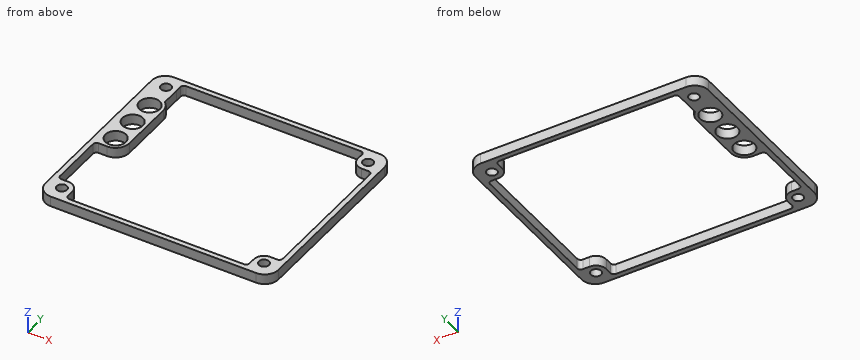
Autodesk Fusion 360 part; units mm, degrees
sketch "Sketch1" plane through (0, 0, 0) normal (0, 0, 1) x (1, 0, 0)
  line L0 (-29.5, 24.5) -> (-35.5, 24.5) construction
  circle A0 centre (29.5, 24.5) radius 1.5
  line L1 (25.5009, -27.5) -> (3.5, -27.5)
  arc A1 (34, 25) -> (30, 29) centre (30, 25) ccw
  circle A2 centre (29.5, -24.5) radius 1.5
  arc A3 (30, -29) -> (34, -25) centre (30, -25) ccw
  line L2 (30, -29) -> (-30, -29)
  arc A4 (-34, -25) -> (-30, -29) centre (-30, -25) ccw
  line L3 (0, -27.5) -> (0.5, -27.5) construction
  line L4 (0.5, -27.5) -> (-25.5, -27.5)
  line L5 (-30, 29) -> (30, 29)
  line L6 (0, 27.5) -> (0.5, 27.5) construction
  circle A5 centre (-29.5, 24.5) radius 1.5
  arc A6 (-30, 29) -> (-34, 25) centre (-30, 25) ccw
  line L7 (0, -27.5) -> (0.5, -27.5) construction
  line L8 (-34, -25) -> (-34, 25)
  circle A7 centre (-29.5, -24.5) radius 1.5
  line L9 (0, -27.5) -> (0.5, -27.5)
  line L10 (34, 25) -> (34, -25)
  line L11 (-29.5, 24.5) -> (-34, 24.5) construction
  line L12 (-34, 24.5) -> (-34, 29) construction
  line L13 (-34, 29) -> (-29.5, 29) construction
  line L14 (-29.5, 29) -> (-29.5, 24.5) construction
  line L15 (-34, 29) -> (-29, 29) construction
  line L16 (-29, 29) -> (-29, 16) construction
  line L17 (-29, 16) -> (-34, 16) construction
  line L18 (-34, 16) -> (-34, 29) construction
  line L19 (-25, 13) -> (-25, 11)
  line L20 (-25, 5) -> (-25, 3)
  line L21 (-25, 13) -> (-25, 16)
  line L22 (-25, 11) -> (-25, 5)
  line L23 (-25, 3) -> (-25, 0)
  line L24 (-26.5, 24.4915) -> (-26.494, 26.6091)
  line L25 (-26.5, 24.4915) -> (-26.5151, 19.1346)
  arc A8 (-25.5, 27.5) -> (-26.4946, 26.3966) centre (-25.5, 26.5) ccw
  line L26 (-30, 27.5) -> (-29, 27.5)
  line L27 (-25.5, 27.5) -> (0.5, 27.5)
  arc A9 (-29, 27.458) -> (-29.5, 27.5) centre (-29.5, 24.5) ccw
  arc A10 (-29, 27.458) -> (-29.5, 27.5) centre (-29.5, 24.5) ccw
  circle A11 centre (-29, 16) radius 3
  circle A12 centre (-29, 8) radius 3
  circle A13 centre (-29, 0) radius 3
  arc A14 (-25, 16) -> (-26.5151, 19.1346) centre (-29, 16) ccw
  arc A15 (-29, -4) -> (-25, 0) centre (-29, 0) ccw
  line L28 (-32.5, -20.5009) -> (-32.5, -4.999)
  line L29 (-29, -3) -> (-29, -4) construction
  line L30 (-29, -4) -> (-31.5, -4)
  line L31 (-29.5, -24.5) -> (-26.5, -24.5) construction
  line L32 (-26.5, -24.5) -> (-26.5, -21.5) construction
  line L33 (-26.5, -21.5) -> (-29.5, -21.5) construction
  line L34 (-29.5, -21.5) -> (-29.5, -24.5) construction
  line L35 (-26.5, -24.5) -> (-26.5, -26.5)
  line L36 (-29.5, -21.5) -> (-31.5, -21.5)
  arc A16 (-26.5, -24.5015) -> (-29.5014, -21.5) centre (-29.5, -24.5) ccw
  arc A17 (-31.5, -4) -> (-32.5, -5.001) centre (-31.5, -5) ccw
  arc A18 (-32.5, -20.4991) -> (-31.5, -21.5) centre (-31.5, -20.5) ccw
  arc A19 (-26.5, -26.5) -> (-25.5, -27.5) centre (-25.5, -26.5) ccw
  line L37 (0.5, 27.5) -> (3.5, 27.5)
  line L38 (3.5, -27.5) -> (0.5, -27.5)
  line L39 (29.5, -24.5) -> (26.5, -24.5) construction
  line L40 (26.5, -24.5) -> (26.5, -21.5) construction
  line L41 (26.5, -21.5) -> (29.5, -21.5) construction
  line L42 (29.5, -21.5) -> (29.5, -24.5) construction
  line L43 (29.5, -21.5) -> (31.5, -21.5)
  line L44 (26.5, -24.5) -> (26.5, -26.5)
  line L45 (32.5, -24.5) -> (32.5, -25)
  arc A20 (29.5014, -21.5) -> (26.5, -24.5015) centre (29.5, -24.5) ccw
  arc A21 (25.4991, -27.5) -> (26.5, -26.5) centre (25.5, -26.5) ccw
  arc A22 (31.5, -21.5) -> (32.5, -20.5) centre (31.5, -20.5) ccw
  line L46 (29.5, 24.5) -> (26.5, 24.5) construction
  line L47 (26.5, 24.5) -> (26.5, 21.5) construction
  line L48 (26.5, 21.5) -> (29.5, 21.5) construction
  line L49 (29.5, 21.5) -> (29.5, 24.5) construction
  line L50 (26.5, 24.5) -> (26.5, 26.5)
  line L51 (29.5, 21.5) -> (31.5, 21.5)
  line L52 (32.5, 25) -> (32.5, 24.5)
  line L53 (32.5, 20.501) -> (32.5, -20.5)
  arc A23 (26.5, 24.5015) -> (29.5014, 21.5) centre (29.5, 24.5) ccw
  line L54 (3.5, 27.5) -> (25.5, 27.5)
  line L55 (29.5, 27.5) -> (30, 27.5)
  arc A24 (26.5, 26.5) -> (25.5, 27.5) centre (25.5, 26.5) ccw
  arc A25 (32.5, 20.499) -> (31.5, 21.5) centre (31.5, 20.5) ccw
  point P0 (-29, 12)
  dimension "d1" = 3
  dimension "d2" = 3
  dimension "d3" = 3
  dimension "d4" = 3
  dimension "d12" = 5
  dimension "d13" = 13
  dimension "d20" = 2
extrude "Extrude1" add sketch "Sketch1" along normal blind 3
equation "gasket_thikness = 3 mm"
equation "d21 = gasket_thikness"
Model file for the job. Use its own axes, mm. Give positions to 0.01 mm unless a question says otherwise; leave off trailing zeros. Order: outer loops, then holes, each group sorted by start corner. A loop starts at its lowest first (then second) coordinate and runs counter-clockwise, first axis right, second up.
1) Wall check: probe 1 along Y at (x, z) = (8, 1.6); probe 2 along X at (y, z) = (-10.5, 0.4); probe 3 along X at (y, z) = (-1, 1.85). Give the ranges that are in metal, low to high.
2) Saw through at D-D, the plane z = 2.55. Count the separate pieces of the cut face and the enclosed holes in it, then the cut area to 3 significant figures.
3) Saw through at B-B, the plane y = -17. Write the cut outline in (x, z).
4) Saw through at C-C, the plane x = 14. Write the cut outline in (y, z).
5) Saw through at A-A, the plane y = 8. Write the cut outline in (x, z), then the cut area to 3 significant figures.
6) Pin check, flat tips, straight feed: pin 1 (0.6 mm diameter, centred on y = -25.5, z = 1, fed in from +X) (3 decimals); pin 2 (0.6 mm diameter, centred on x = -30.5, z = 2, fed in from +Y) (3 decimals). Stop position of each tip, or through.
Computed:
1. probe 1: y = -29 to -27.5, 27.5 to 29
1. probe 2: x = -34 to -32.5, 32.5 to 34
1. probe 3: x = -34 to -31.83, -26.17 to -25.13, 32.5 to 34
2. separate pieces: 1
2. enclosed holes: 8
2. area: 565 mm2
3. outline: (-34, 0) - (-32.5, 0) - (-32.5, 3) - (-34, 3) - close; (32.5, 0) - (34, 0) - (34, 3) - (32.5, 3) - close
4. outline: (-29, 0) - (-27.5, 0) - (-27.5, 3) - (-29, 3) - close; (27.5, 0) - (29, 0) - (29, 3) - (27.5, 3) - close
5. outline: (-34, 0) - (-32, 0) - (-32, 3) - (-34, 3) - close; (-26, 0) - (-25, 0) - (-25, 3) - (-26, 3) - close; (32.5, 0) - (34, 0) - (34, 3) - (32.5, 3) - close
5. area: 13.5 mm2
6. pin 1: stops at x = 33.995
6. pin 2: stops at y = 28.995
